Autodesk Inventor part; units mm, degrees
ref_plane "YZ Plane" through (0, 0, 0) normal (1, 0, 0) x (0, 1, 0)
ref_plane "XZ Plane" through (0, 0, 0) normal (0, 1, 0) x (-1, 0, 0)
ref_plane "XY Plane" through (0, 0, 0) normal (0, 0, 1) x (1, 0, 0)
sketch "Sketch1" plane through (0, 0, 0) normal (0, 0, 1) x (1, 0, 0)
  circle A0 centre (4.25, 3.95) radius 1.4
  circle A1 centre (-4.25, 3.95) radius 1.4
  circle A2 centre (-4.25, -3.95) radius 1.4
  circle A3 centre (4.25, -3.95) radius 1.4
  line L0 (-5, 7) -> (5, 7)
  line L1 (7, 5) -> (7, -5)
  line L2 (5, -7) -> (-5, -7)
  line L3 (-7, -5) -> (-7, 5)
  arc A4 (-5, 7) -> (-7, 5) centre (-5, 5) ccw
  arc A5 (7, 5) -> (5, 7) centre (5, 5) ccw
  arc A6 (5, -7) -> (7, -5) centre (5, -5) ccw
  arc A7 (-7, -5) -> (-5, -7) centre (-5, -5) ccw
  circle A8 centre (-4.25, 3.95) radius 2.25
  circle A9 centre (4.25, 3.95) radius 2.25
  circle A10 centre (4.25, -3.95) radius 2.25
  circle A11 centre (-4.25, -3.95) radius 2.25
  point P0 (0, 0)
extrude "Extrusion1" add sketch "Sketch1" along normal blind 1 contours A8 | A9 | A10 | A11
extrude "Extrusion2" add sketch "Sketch1" against normal blind 10 contours L0 A5 L1 A6 L2 A7 L3 A4 | A8 | A9 | A10 | A11
sketch "Sketch2" plane through (-7, -5, 0) normal (-1, 0, 0) x (0, 0, 1)
  circle A0 centre (-5, 5) radius 1.45
  point P0 (0, 5)
extrude "Extrusion3" cut sketch "Sketch2" against normal blind 20
chamfer "Chamfer1" distance 0.5 angle 45 2 edges at (-7, 0, -6.45) (7, 0, -6.45)
sketch "Sketch3" plane through (0, 0, -10) normal (0, 0, -1) x (-1, 0, 0)
  circle A0 centre (4.25, -3.95) radius 1.4
  circle A1 centre (-4.25, -3.95) radius 1.4
  circle A2 centre (-4.25, 3.95) radius 1.4
  circle A3 centre (4.25, 3.95) radius 1.4
  point P0 (0, 0)
extrude "Extrusion4" add sketch "Sketch3" against normal blind 6
chamfer "Chamfer2" distance 0.2 angle 45 8 edges at (2.85, -3.95, 1) (-5.65, -3.95, 1) (2.85, 3.95, 1) (-5.65, 3.95, 1) (2, -3.95, 1) (-6.5, -3.95, 1) (-6.5, 3.95, 1) (2, 3.95, 1)
sketch "Sketch4" plane through (-4.25, 3.95, 1) normal (0, 0, 1) x (1, 0, 0)
  circle A0 centre (0, 0) radius 3.95
  circle A1 centre (0, -7.9) radius 3.95
  circle A2 centre (8.5, -7.9) radius 3.95
  circle A3 centre (8.5, 0) radius 3.95
  point P0 (4.25, -3.95)
  point P1 (8.5, -3.95)
  point P2 (0, -3.95)
extrude "Extrusion5" add sketch "Sketch4" along normal blind 4
sketch "Sketch5" plane through (-7, -5, 0) normal (-1, 0, 0) x (0, 0, 1)
  line L0 (-0.5, -2.9) -> (6.5, -2.9)
  line L1 (6.5, -2.9) -> (6.5, 12.9)
  line L2 (6.5, 12.9) -> (-0.5, 12.9)
  line L3 (-0.5, 14.9) -> (8.5, 14.9)
  line L4 (8.5, 14.9) -> (8.5, -4.9)
  line L5 (8.5, -4.9) -> (-0.5, -4.9)
  line L6 (-0.5, 12.9) -> (-0.5, 14.9)
  line L7 (-0.5, -4.9) -> (-0.5, -2.9)
  circle A0 centre (-5, 5) radius 1.45
  circle A1 centre (-5, 5) radius 1.45
sketch "Sketch6" plane through (0, 0, -10) normal (0, 0, -1) x (-1, 0, 0)
  line L0 (7, -1.95) -> (7, 1.95)
  line L1 (7, 0) -> (-7, 0)
  line L2 (-7, 0) -> (-7, -17)
  line L3 (-7, -17) -> (7, -17)
  line L4 (7, -17) -> (7, 0)
  line L5 (-5, -7) -> (5, -7)
  arc A0 (-7, -5) -> (-5, -7) centre (-5, -5) ccw
  arc A1 (5, -7) -> (7, -5) centre (5, -5) ccw
  point P0 (0, 0)
  dimension "d37" = 17
extrude "Extrusion6" add sketch "Sketch6" against normal blind 8 contours L4 L3 L2 A0 L5 A1
sketch "Sketch7" plane through (0, 0, -2) normal (0, 0, 1) x (1, 0, 0)
  line L0 (-5, -7) -> (5, -7)
  line L1 (0, -7) -> (0, -11)
  line L2 (7, 5) -> (7, -17)
  line L3 (-7, -17) -> (-7, 5)
  line L4 (7, -11) -> (-7, -11)
  line L5 (-7, -11) -> (-7, -17)
  line L6 (-7, -17) -> (7, -17)
  line L7 (7, -17) -> (7, -11)
  point P0 (0, 0)
extrude "Extrusion7" add sketch "Sketch7" along normal blind 12
sketch "Sketch8" plane through (0, 0, -10) normal (0, 0, -1) x (-1, 0, 0)
  arc A0 (-5, 7) -> (-7, 5) centre (-5, 5) ccw
  line L0 (7, 5) -> (7, 19.5)
  line L1 (7, 19.5) -> (-7, 19.5)
  line L2 (-7, 19.5) -> (-7, 5)
  arc A1 (7, 5) -> (5, 7) centre (5, 5) ccw
  line L3 (5, 7) -> (-5, 7)
  point P0 (0, 0)
extrude "Extrusion8" add sketch "Sketch8" against normal blind 3.5
sketch "Sketch9" plane through (0, 0, 10) normal (0, 0, 1) x (1, 0, 0)
  line L0 (7, -11) -> (-7, -11)
  line L1 (7, 19.5) -> (7, -17)
  line L2 (-7, -11) -> (7, -11)
  line L3 (7, -11) -> (7, -11.4)
  line L4 (7, -11.4) -> (-7, -11.4)
  line L5 (-7, -11.4) -> (-7, -11)
  point P0 (0, 0)
  dimension "d47" = 0.4
extrude "Extrusion9" cut sketch "Sketch9" against normal up to surface (12 mm away)
sketch "Sketch10" plane through (0, 0, -6.5) normal (0, 0, 1) x (1, 0, 0)
  line L0 (-7, 19.5) -> (7, 19.5)
  line L1 (0, 19.5) -> (0, 9.5)
  circle A0 centre (0, 9.5) radius 0.9
  circle A1 centre (0, 14.5) radius 0.9
  point P0 (0, 0)
  dimension "d50" = 10
  dimension "d51" = 1.8
  dimension "d52" = 1.8
extrude "Extrusion10" cut sketch "Sketch10" against normal blind 10
fillet "Fillet1" radius 2 2 edges at (-7, 19.5, -8.25) (7, 19.5, -8.25)
sketch "Sketch12" plane through (0, 0, -10) normal (0, 0, -1) x (-1, 0, 0)
  line L0 (7, -17) -> (-7, -17)
  line L1 (7, -17) -> (2, -17)
  line L2 (-7, -17) -> (-2, -17)
  circle A0 centre (4.5, -20) radius 1
  circle A1 centre (4.5, -20) radius 2.5
  circle A2 centre (-4.5, -20) radius 1
  circle A3 centre (-4.5, -20) radius 2.5
  line L3 (7, -17) -> (7, -20)
  line L4 (-7, -17) -> (-7, -20)
  line L5 (-4.5, -22.5) -> (4.5, -22.5)
  point P0 (0, 0)
  dimension "d57" = 5
extrude "Extrusion11" add sketch "Sketch12" against normal blind 3
sketch "Sketch13" plane through (0, 0, 10) normal (0, 0, 1) x (1, 0, 0)
  line L0 (7, -20) -> (7, -17)
  line L1 (-7, -17) -> (7, -17)
  line L2 (-7, -17) -> (-7, -20)
  arc A0 (-7, -20) -> (-4.5, -22.5) centre (-4.5, -20) ccw
  line L3 (-4.5, -22.5) -> (4.5, -22.5)
  arc A1 (4.5, -22.5) -> (7, -20) centre (4.5, -20) ccw
  circle A2 centre (-4.5, -20) radius 1
  circle A3 centre (4.5, -20) radius 1
  line L4 (7, -11.4) -> (-7, -11.4)
  line L5 (-7, -11.4) -> (-7, -17)
  line L6 (-7, -17) -> (7, -17)
  line L7 (7, -17) -> (7, -11.4)
  circle A4 centre (4.5, -14.2) radius 0.9
  circle A5 centre (-4.5, -14.2) radius 0.9
  point P0 (0, 0)
extrude "Extrusion12" cut sketch "Sketch13" against normal blind 3 contours L1 L5 L4 L7 | A4 | A5
extrude "Extrusion13" cut sketch "Sketch13" against normal blind 12 contours A4 | A5
fillet "Fillet2" radius 1 1 edges at (0, -11.4, -2)
sketch "Sketch14" plane through (0, 0, -10) normal (0, 0, -1) x (-1, 0, 0)
  circle A0 centre (-4.5, -20) radius 1
  circle A1 centre (4.5, -20) radius 1
  circle A2 centre (0, -27.2111) radius 6.5
  point P0 (0, 0)
extrude "Extrusion14" cut sketch "Sketch14" against normal blind 12 contours A2
fillet "Fillet3" radius 1 2 edges at (-4.4783, -22.5, -8.5) (4.4783, -22.5, -8.5)
sketch "Sketch16" plane through (0, 0, -10) normal (0, 0, -1) x (-1, 0, 0)
  line L0 (-7, -17) -> (7, -17)
  line L1 (-7, -17) -> (-1, -17)
  line L2 (-1, -17) -> (-1, -11)
  line L3 (-1, -11) -> (-7, -11)
  line L4 (-7, -11) -> (-7, -17)
  line L5 (-5, 19.5) -> (-0.9, 19.5)
  line L6 (-0.9, 19.5) -> (-0.9, 13)
  line L7 (-0.9, 13) -> (-7, 13)
  line L8 (-7, 13) -> (-7, 17.5)
  line L9 (-7, 17.5) -> (-7, -20)
  line L10 (-0.9, 13) -> (-7, 13)
  line L11 (-7, 13) -> (-7, 15)
  line L12 (-7, 15) -> (-0.9, 15)
  line L13 (-0.9, 15) -> (-0.9, 13)
  line L14 (-7, -11) -> (-1, -11)
  line L15 (-1, -11) -> (-1, -13)
  line L16 (-1, -13) -> (-7, -13)
  line L17 (-7, -13) -> (-7, -11)
  circle A0 centre (-3.95, 17.25) radius 0.9
  circle A1 centre (-4, -15) radius 0.9
  arc A2 (-5, 19.5) -> (-7, 17.5) centre (-5, 17.5) ccw
  point P0 (0, 0)
  dimension "d83" = 2
extrude "Extrusion15" cut sketch "Sketch16" against normal blind 6 contours A0 | A1
chamfer "Chamfer3" distance 0.4 angle 45 6 edges at (4.9, -15, -10) (4.85, 17.25, -10) (5.5, -20, -10) (-3.5, -20, -10) (5.5, -20, -7) (-3.5, -20, -7)
sketch "Sketch17" plane through (-4.25, 3.95, 5) normal (0, 0, 1) x (1, 0, 0)
  circle A0 centre (0, 0) radius 3.95
  circle A1 centre (8.5, 0) radius 3.95
  circle A2 centre (8.5, -7.9) radius 3.95
  circle A3 centre (0, -7.9) radius 3.95
  point P0 (4.25, -3.95)
  point P1 (0, -3.95)
  point P2 (8.5, -3.95)
  point P3 (8.5, -3.95)
  point P4 (0, -3.95)
  point P5 (8.5, -3.95)
  point P6 (0, -3.95)
extrude "Extrusion16" cut sketch "Sketch17" against normal blind 4
sketch "Sketch18" plane through (0, 0, 0) normal (0, 0, 1) x (1, 0, 0)
  line L0 (7, -10.4) -> (-7, -10.4)
  line L1 (7, -10.4) -> (7, -5)
  arc A0 (5, -7) -> (7, -5) centre (5, -5) ccw
  line L2 (-5, -7) -> (5, -7)
  arc A1 (-7, -5) -> (-5, -7) centre (-5, -5) ccw
  line L3 (-7, -5) -> (-7, -10.4)
  line L4 (-7, -10.4) -> (-7, -11.4)
  line L5 (-7, -11.4) -> (7, -11.4)
  line L6 (7, -11.4) -> (7, -10.4)
  line L7 (7, -10.4) -> (-7, -10.4)
  circle A2 centre (-4.5, -14.2) radius 0.9
  circle A3 centre (4.5, -14.2) radius 0.9
  line L8 (7, -17) -> (-7, -17)
  line L9 (7, -11.4) -> (7, -17)
  line L10 (-7, -11.4) -> (7, -11.4)
  line L11 (-7, -17) -> (-7, -11.4)
  circle A4 centre (4.5, -20) radius 1.4
  arc A5 (4.1777, -22.2315) -> (5.0341, -22.4423) centre (4.8204, -21.4654) ccw
  arc A6 (5.0341, -22.4423) -> (7, -20) centre (4.5, -20) ccw
  line L12 (7, -20) -> (7, -17)
  line L13 (-7, -17) -> (7, -17)
  line L14 (-7, -17) -> (-7, -20)
  arc A7 (-7, -20) -> (-5.0341, -22.4423) centre (-4.5, -20) ccw
  arc A8 (-5.0341, -22.4423) -> (-4.1777, -22.2315) centre (-4.8204, -21.4654) ccw
  arc A9 (4.1777, -22.2315) -> (-4.1777, -22.2315) centre (0, -27.2111) ccw
  circle A10 centre (-4.5, -20) radius 1.4
  line L15 (-7, -17) -> (-7, -11.4)
  line L16 (7, -11.4) -> (7, -17)
  point P0 (0, 0)
extrude "Extrusion17" cut sketch "Sketch18" along normal mid plane 30 contours L6 L5 L4 L0 | L0 L3 A1 L2 A0 L1 | L9 L8 L11 L5 | L12 A6 A5 A9 A8 A7 L14 L8 | A2 | A3 | A4 | A10
sketch "Sketch19" plane through (0, 0, -10) normal (0, 0, -1) x (-1, 0, 0)
  arc A0 (5, -7) -> (7, -5) centre (5, -5) ccw
  line L0 (7, -5) -> (-7, -5)
  line L1 (-7, -5) -> (-7, -17.5)
  line L2 (-5, -19.5) -> (5, -19.5)
  line L3 (7, -17.5) -> (7, -5)
  arc A1 (5, -19.5) -> (7, -17.5) centre (5, -17.5) ccw
  arc A2 (-7, -17.5) -> (-5, -19.5) centre (-5, -17.5) ccw
  point P0 (0, 0)
  dimension "d98" = 2
extrude "Extrusion18" add sketch "Sketch19" against normal up to surface (3.5 mm away)
sketch "Sketch20" plane through (0, 0, -10) normal (0, 0, -1) x (-1, 0, 0)
  circle A0 centre (-3.95, 17.25) radius 1.3
  circle A1 centre (-3.95, 17.25) radius 1.3
  point P0 (0, 0)
extrude "Extrusion19" add sketch "Sketch20" against normal blind 3.5
sketch "Sketch21" plane through (0, 0, -10) normal (0, 0, -1) x (-1, 0, 0)
  arc A0 (-5, 19.5) -> (-7, 17.5) centre (-5, 17.5) ccw
  arc A1 (5, -19.5) -> (7, -17.5) centre (5, -17.5) ccw
  circle A2 centre (-4, -16.5) radius 0.9
  circle A3 centre (4, -16.5) radius 0.9
  circle A4 centre (4, 16.5) radius 0.9
  circle A5 centre (-4, 16.5) radius 0.9
extrude "Extrusion20" cut sketch "Sketch21" against normal blind 3.5
sketch "Sketch22" plane through (-7, -5, 0) normal (-1, 0, 0) x (0, 0, 1)
  circle A0 centre (-5, 5) radius 1.45
  circle A1 centre (-5, 5) radius 1.525
  point P0 (0, 5)
  dimension "d110" = 3.05
extrude "Extrusion21" cut sketch "Sketch22" against normal blind 20
sketch "Sketch23" plane through (0, 0, -10) normal (0, 0, -1) x (-1, 0, 0)
  circle A0 centre (-4, -16.5) radius 0.9
  circle A1 centre (4, 16.5) radius 0.9
  circle A2 centre (4, -16.5) radius 0.9
  circle A3 centre (-4, 16.5) radius 0.9
  line L0 (7, -17.5) -> (7, 17.5)
  arc A4 (7, 17.5) -> (5, 19.5) centre (5, 17.5) ccw
  line L1 (5, 19.5) -> (-5, 19.5)
  arc A5 (-5, 19.5) -> (-7, 17.5) centre (-5, 17.5) ccw
  line L2 (-7, 17.5) -> (-7, -17.5)
  arc A6 (-7, -17.5) -> (-5, -19.5) centre (-5, -17.5) ccw
  line L3 (-5, -19.5) -> (5, -19.5)
  arc A7 (5, -19.5) -> (7, -17.5) centre (5, -17.5) ccw
  circle A8 centre (0, 14.5) radius 0.9
  circle A9 centre (0, 9.5) radius 0.9
  point P0 (0, 0)
extrude "Extrusion22" add sketch "Sketch23" along normal blind 10
properties part number "slider" material "Steel"
Here's how the part is built. I have some questions about the finished solid (model axes, mm). A direction names the side the tool comes from. Coordinates: 2 decimals unless noted, no trailing zeros. Loops run counter-clockwise (first coordinate to the right, second up) from the corner with the lowest first, then second, coordinate; pieces in that order, holes last. Notation, with made-up numbers: (83.5, -26) - (108.5, -26) arc R22 cw to (108.5, 5) - close; hole circle Ø8 at (-9, -26). An arc over 180 degrees is marked (long way). Return JSON: item names as keys, results as strings. Group by question number.
Item 1: Will these pins go through, and if not, where does the flat tip stop? P1, Ø5, axis at x = -0.5, z = -3, coming from the +Y side; P2, Ø1.4, axis at x = 0, y = 14.5, coming from the +Z side; P3, Ø3, axis at x = -2, z = -3, coming from the -Y side; P4, Ø2, axis at x = 4.5, y = -3.5, coming from the +Z side.
Item 2: We'd pull the mould along X, two halves only. Please class faces 1 (the face through (7, 0, -12)), 2 (the face through (-2.104, 3.274, 0.394)), 3 (the face through (-6.4, 18.93, -13.16)), 4 (the face through (4.12, -17.39, -13.16)): +X half, -X half, draft (parallel to the pull), parting line (faces both ways), or undercut.
Item 3: If we section it at D-D on x = 0.5: Write out the boundary of the cut face in (y, z) (3 decimals).
Item 4: On a 3-axis mill with a long thin cutter (end or side, diameter ignored), from which of +Z, -Z, +X, -X, +Y, -Y can I reach the whole of each face in a straight line? I mean faces 5 (the face through (-3.88, 15.61, -13.16)), 6 (the face through (5.288, -1.954, 0.394)). Say none if no direction works.
Item 5: I need wall thicknesses on line 1 (X direction, y = -3.95, z = -2.1); line 2 (Y direction, x = 0, z = -9.25); line 3 (Y direction, x = -4.25, z = -3). Which ranges of each line are inside material? Lowest first, please. Write a range as from..to.
Item 6: If we section it at C-C on z = -5: Write out the boundary of the cut face in (x, y) (3 decimals), and give its area (3 significant figures).
Item 7: If we section it at A-A on y = -16.5: Write out the boundary of the cut face in (x, z), and give its area (3 significant figures).
Item 8: If we section it at B-B on z = -17.5: Write out the boundary of the cut face in (x, y), and give its area (3 significant figures).
Calculated:
{
 "1": {"P1": "stops at y = 7", "P2": "passes through", "P3": "stops at y = -7", "P4": "stops at z = 0.91"},
 "2": {"face 1": "+X half", "face 2": "undercut", "face 3": "-X half", "face 4": "undercut"},
 "3": {"outline": "(-19.5, -20) - (8.752, -20) - (8.752, -6.5) - (7, -6.5) - (7, 0) - (-7, 0) - (-7, -6.5) - (-19.5, -6.5) - close; (10.248, -20) - (13.752, -20) - (13.752, -6.5) - (10.248, -6.5) - close; (15.248, -20) - (19.5, -20) - (19.5, -6.5) - (15.248, -6.5) - close; hole circle Ø3.05 at (0, -5)"},
 "4": {"face 5": "+Z, -Z", "face 6": "+Z"},
 "5": {"line 1": "x = -7..-5.65, -2.85..2.85, 5.65..7", "line 2": "y = -19.5..8.6, 10.4..13.6, 15.4..19.5", "line 3": "y = -7..-5.35, -2.55..2.55, 5.35..7"},
 "6": {"outline": "(-7, -5) arc R2 ccw to (-5, -7) - (5, -7) arc R2 ccw to (7, -5) - (7, -1.95) - (6.575, -1.525) - (-6.575, -1.525) - (-7, -1.95) - close; (-7, 1.95) - (-6.575, 1.525) - (6.575, 1.525) - (7, 1.95) - (7, 5) arc R2 ccw to (5, 7) - (-5, 7) arc R2 ccw to (-7, 5) - close", "area": "150 mm^2"},
 "7": {"outline": "(-7, -20) - (-4.9, -20) - (-4.9, -6.5) - (-7, -6.5) - close; (-3.1, -20) - (3.1, -20) - (3.1, -6.5) - (-3.1, -6.5) - close; (4.9, -20) - (7, -20) - (7, -6.5) - (4.9, -6.5) - close", "area": "140 mm^2"},
 "8": {"outline": "(-7, -17.5) arc R2 ccw to (-5, -19.5) - (5, -19.5) arc R2 ccw to (7, -17.5) - (7, 17.5) arc R2 ccw to (5, 19.5) - (-5, 19.5) arc R2 ccw to (-7, 17.5) - close; hole circle Ø1.8 at (-4, -16.5); hole circle Ø1.8 at (-4, 16.5); hole circle Ø1.8 at (0, 9.5); hole circle Ø1.8 at (0, 14.5); hole circle Ø1.8 at (4, -16.5); hole circle Ø1.8 at (4, 16.5)", "area": "527 mm^2"}
}
